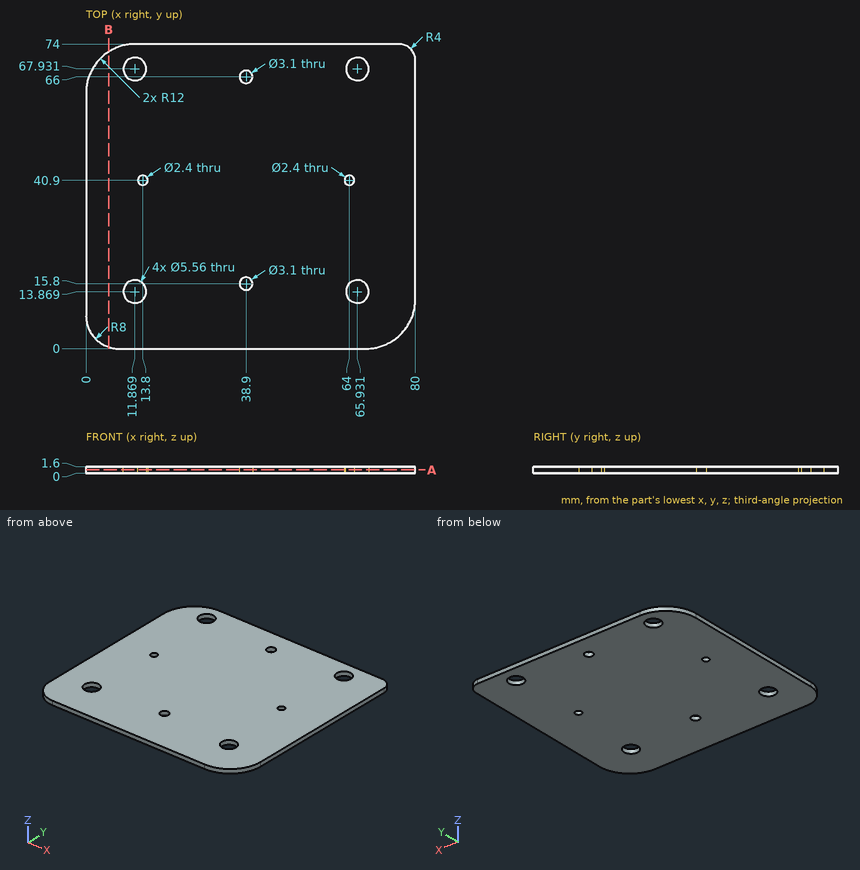
Study the drawing (mm; zero at the part's minimum x, y, z) and answer. Coordinates: 2 decimals unless noted, no trailing zeros. Order: outer loops, then holes, each group sorted by start corner. A loop starts at its lowest first (then second) coordinate and runs counter-clockwise, first axis right, second up. Notation, with made-up numbers: M -39.5,2.5 L 14.5,2.5 A24 cw 14.5,13.5 Z; hole C 47,48 d5. An arc over 180 degrees is marked long. Answer as a JSON object with one key per item and string values. Group by question number.
1. Section A-A on z = 0.8 is taken. State how many separate pieces and enclosed holes the cut face has, then the cut area to 3 significant figures.
2. Section B-B on x = 5.5 is taken. Write down the section's boundary in (y, z).
3. Straight lines are drawn through the part: line 1 (Y direction, x = 66, z = 0.45); line 2 (Y direction, x = 64, z = 1.15); line 3 (Y direction, x = 74, z = 0.5). For each, find the intervals that lie inside material, in ascending order.
Values follow:
{
 "1": {"separate pieces": "1", "enclosed holes": "8", "area": "5,720 mm2"},
 "2": {"outline": "M 0.4,0 L 72.09,0 L 72.09,1.6 L 0.4,1.6 Z"},
 "3": {"line 1": "0 to 11.09, 16.65 to 65.15, 70.71 to 74", "line 2": "0 to 11.87, 15.87 to 39.7, 42.1 to 65.93, 69.93 to 74", "line 3": "1.61 to 74"}
}
